Could you check a few things on this drawing? It's one solid part, dimensions in mm from its lowest x, y, z. Round coordinates to 2 decimals unless told otherwise and drop trailing zeros. Write each loop counter-clockwise with the first axis right and the second up, starting at its lowest first coordinate (ties: lowest second). Pieces come first, ordered by that corner, then holes. Notation, with made-up numbers: (70.5, 31.25) - (99.5, 31.25) arc R17 cw to (99.5, 44.25) - close; hole circle Ø4 at (-21, 63). An arc over 180 degrees is marked (long way). Put each result on its own line as item: value.
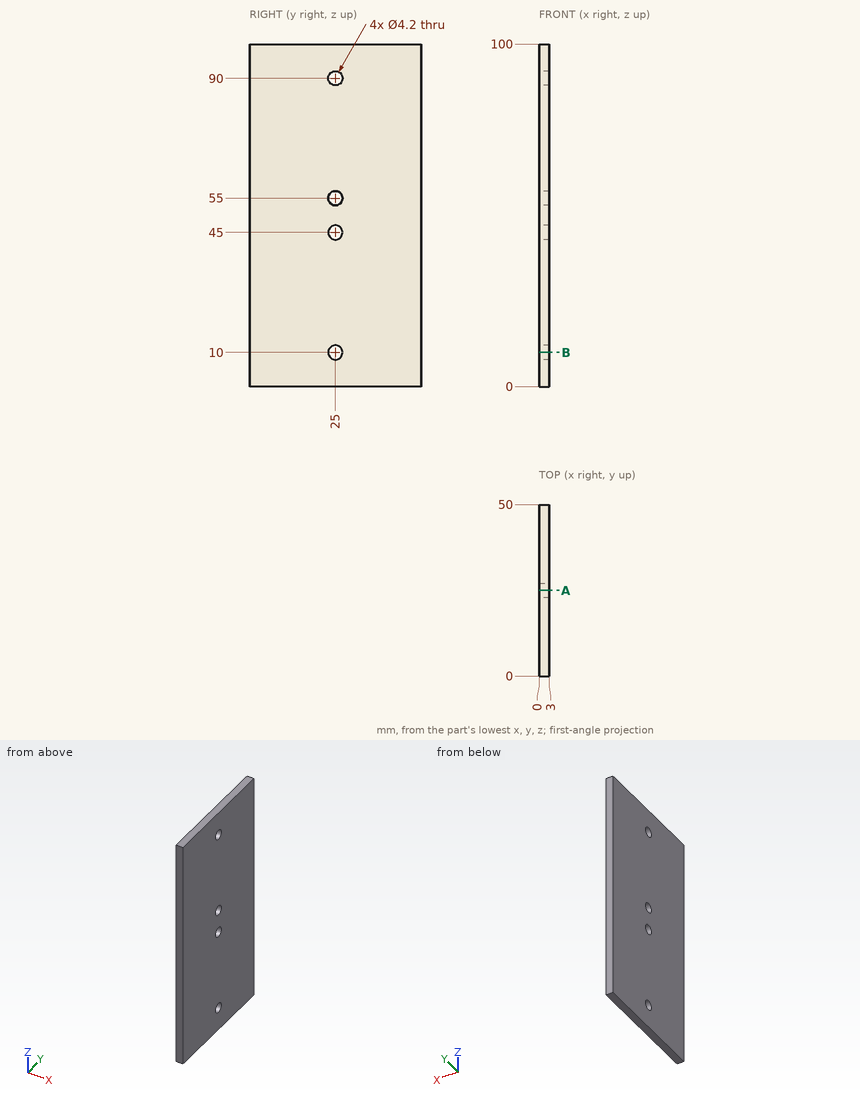
(1) I'm going to push a flat-ended pin straight in: pin 1 (4 mm diameter, centred on y = 25, z = 45, fed in from +X). Where does the tip first touch, or does it pass through?
Values found:
pin 1: passes through
(2) Imagine slicing it at A-A, the plane y = 25. List the corners of the cut face in (x, z) for me.
Values found:
outline: (0, 0) - (3, 0) - (3, 7.9) - (0, 7.9) - close; (0, 12.1) - (3, 12.1) - (3, 42.9) - (0, 42.9) - close; (0, 47.1) - (3, 47.1) - (3, 52.9) - (0, 52.9) - close; (0, 57.1) - (3, 57.1) - (3, 87.9) - (0, 87.9) - close; (0, 92.1) - (3, 92.1) - (3, 100) - (0, 100) - close
(3) Imagine slicing it at B-B, the plane z = 10. List the corners of the cut face in (x, y) for me.
Values found:
outline: (0, 0) - (3, 0) - (3, 22.9) - (0, 22.9) - close; (0, 27.1) - (3, 27.1) - (3, 50) - (0, 50) - close
(4) Please list where these lines run through material, in increasing order: probe 1 along Z at (x, y) = (2, 25); probe 2 along Y at (x, z) = (1.5, 90); probe 3 along Z at (x, y) = (2.15, 24). Write a range as from..to.
Values found:
probe 1: z = 0..7.9, 12.1..42.9, 47.1..52.9, 57.1..87.9, 92.1..100
probe 2: y = 0..22.9, 27.1..50
probe 3: z = 0..8.15, 11.85..43.15, 46.85..53.15, 56.85..88.15, 91.85..100
